Part model, mm, in its own coordinate system. Face numbers are marked on the shaded views. A direction names the side the tool comes from. Round coordinates to 2 decimals unless told otherwise and drop trailing zeros. Write each loop counter-clockwise with the first axis right and the second up, starting at its lowest first coordinate (ties: lowest second). Pieces come first, ordered by that corner, then holes. Notation, with made-up numbers: M -37,33.5 L 15,33.5 A15 ccw 15,45.5 Z; hole C -2.75,29 d4. An arc over 180 degrees is marked long. Use one line per item in the form item = value. Start each with the question number.
Item 1: Which spindle directions (+Z, -Z, +X, -X, +Y, -Y) get a long thin tool onto all of the face, cutting with end or side? Do the marked faces 1, 2, 3 and 4. Say none if no direction does.
Item 2: Cut at A-A, the plane z = 1.5. State how many separate pieces and enclosed holes the cut face has, then the cut area to 3 significant figures.
Item 3: Cut at D-D, the plane x = -15. Give the cut face in (y, z).
Item 4: Probe L1, parallel to X at y = -1.5, z = 0.5; L2, parallel to Y at x = 9.5, z = 6.75; L3, parallel to Y at x = -32, z = 2.75. List the from-to ranges inside material, lowest first.
Item 5: Mould opens along X. For the marked faces 5, 6, 7 and 8 say: +X half, -X half, draft (parallel to the pull), parting line (faces both ways), or undercut.
Item 6: Flat gauge pins, fed straight in: pin 1 Ø19.5 at (x, y) = (0, 0) entering from +Z; pin 2 Ø1 at (x, z) = (-10.5, 7.5) entering from -Y; pin 3 Ø6 at (x, z) = (19, 5.5) entering from +Y. Where does each tip first touch, or does it go through?
Item 7: Cut at C-C, the plane x = -35.5. Give the cut face in (y, z), then the cut area to 3 significant figures.
Item 8: Cut at B-B, the plane y = -27. Give the cut face in (x, z).
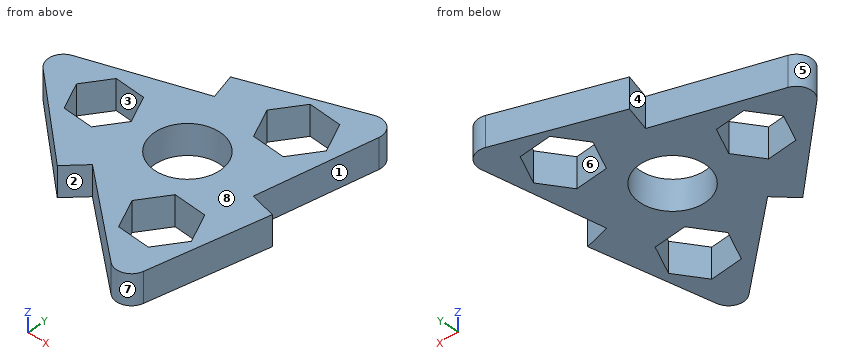
from build123d import *

# Parameters (mm, degrees)
F0_R     = 10.9
F1_DEPTH = 10
F2_R     = 5


with BuildPart() as f1:
    # F0 (on Top) → F1 (new body)
    with BuildSketch(Plane.XY):
        Polygon((-9.80383, 20.148403), (-54.278841, 5.529257), (-19.380784, -25.677659), (-13.404791, -19.551069), (22.350943, -49.771483), (31.927897, -3.945421), (23.634117, -1.833355), (31.927897, 44.242227), (-12.121617, 28.38706), align=None)
        Polygon((24.612059, -24.987273), (18.487568, -33.808305), (7.786085, -32.914856), (3.209092, -23.200375), (9.333583, -14.379343), (20.035067, -15.272792), align=None, mode=Mode.SUBTRACT)
        Polygon((-33.468196, -8.133371), (-37.68838, 0.823798), (-32.041335, 8.957169), (-22.174107, 8.133371), (-17.953923, -0.823798), (-23.600968, -8.957169), align=None, mode=Mode.SUBTRACT)
        Circle(F0_R, mode=Mode.SUBTRACT)
        Polygon((9.333583, 33.808305), (20.035067, 32.914856), (24.612059, 23.200375), (18.487568, 14.379343), (7.786085, 15.272792), (3.209092, 24.987273), align=None, mode=Mode.SUBTRACT)
    extrude(amount=F1_DEPTH)

    # F2
    f2_edges = [f1.edges().sort_by_distance(p)[0] for p in [
        (22.350943, -49.771483, 5),
        (31.927897, 44.242227, 5),
        (-54.278841, 5.529257, 5),
    ]]
    fillet(f2_edges, radius=F2_R)


solid = f1.part
Model answer:
q1.face_1 = +Z, -Z, +X
q1.face_2 = +Z, -Z, -Y
q1.face_3 = +Z, -Z
q1.face_4 = +Z, -Z, -X
q2.separate_pieces = 1
q2.enclosed_holes = 4
q2.area = 2,620 mm²
q3.outline = M -21.19,0 L 18.44,0 L 18.44,10 L -21.19,10 Z
q4.L1 = -46.42 to -36.59, -18.42 to -10.8, 10.8 to 23.69
q4.L2 = -38.91 to -33.06, -14.39 to -5.34, 5.34 to 15.13, 33.79 to 36.17
q4.L3 = -14.39 to -8.26, 8.95 to 12.85
q5.face_5 = -X half
q5.face_6 = undercut
q5.face_7 = parting line
q5.face_8 = draft
q6.pin_1 = through
q6.pin_2 = -22.43
q6.pin_3 = 40.67
q7.outline = M -11.26,0 L -3.82,0 L -3.82,10 L -11.26,10 Z; M 3.98,0 L 11.7,0 L 11.7,10 L 3.98,10 Z
q7.area = 152 mm²
q8.outline = M -4.59,0 L 5,0 L 5,10 L -4.59,10 Z; M 23.21,0 L 27.11,0 L 27.11,10 L 23.21,10 Z
